```python
from build123d import *

# Parameters (mm, degrees)
Y_KSEKLIK_EKSTR_ZYON1_DEPTH = 2
Y_KSEKLIK_EKSTR_ZYON2_DEPTH = 60
IZIM3_R                     = 3.1
KES_EKSTR_ZYON1_DEPTH       = 10


with BuildPart() as part:
    # Çizim1 → Yükseklik-Ekstrüzyon1 (new body)
    with BuildSketch(Plane(origin=(0, 0, 0), x_dir=(1, 0, 0), z_dir=(0, 1, 0))):
        with BuildLine():
            Line((10, 0), (90, 0))
            ThreePointArc((90, 0), (97.071067812, 2.928932188), (100, 10))
            Line((100, 10), (100, 50))
            ThreePointArc((100, 50), (97.071067812, 57.071067812), (90, 60))
            Line((90, 60), (10, 60))
            ThreePointArc((10, 60), (2.928932188, 57.071067812), (0, 50))
            Line((0, 50), (0, 10))
            ThreePointArc((0, 10), (2.928932188, 2.928932188), (10, 0))
        make_face()
    extrude(amount=Y_KSEKLIK_EKSTR_ZYON1_DEPTH)

    # Çizim2 → Yükseklik-Ekstrüzyon2 (add)
    with BuildSketch(Plane(origin=(0, 2, 0), x_dir=(1, 0, 0), z_dir=(0, 1, 0))):
        with BuildLine():
            Line((100, 10), (100, 50))
            ThreePointArc((100, 50), (97.071067812, 57.071067812), (90, 60))
            Line((90, 60), (10, 60))
            ThreePointArc((10, 60), (2.928932188, 57.071067812), (0, 50))
            Line((0, 50), (0, 10))
            ThreePointArc((0, 10), (2.928932188, 2.928932188), (10, 0))
            Line((10, 0), (90, 0))
            ThreePointArc((90, 0), (97.071067812, 2.928932188), (100, 10))
        make_face()
        Polygon((12, 2), (88, 2), (98, 12), (98, 48), (88, 58), (12, 58), (2, 48), (2, 12), align=None, mode=Mode.SUBTRACT)
    extrude(amount=Y_KSEKLIK_EKSTR_ZYON2_DEPTH)

    # Çizim3 → Kes-Ekstrüzyon1 (cut)
    with BuildSketch(Plane.XY):
        with Locations((20, 37)):
            Circle(IZIM3_R)
        with BuildLine():
            Line((76.4, 2), (83.4, 2))
            ThreePointArc((83.4, 2), (84.107106781, 2.292893219), (84.4, 3))
            Line((84.4, 3), (84.4, 6))
            ThreePointArc((84.4, 6), (84.107106781, 6.707106781), (83.4, 7))
            Line((83.4, 7), (76.4, 7))
            ThreePointArc((76.4, 7), (75.692893219, 6.707106781), (75.4, 6))
            Line((75.4, 6), (75.4, 3))
            ThreePointArc((75.4, 3), (75.692893219, 2.292893219), (76.4, 2))
        make_face()
    extrude(amount=-KES_EKSTR_ZYON1_DEPTH, mode=Mode.SUBTRACT)


solid = part.part
```
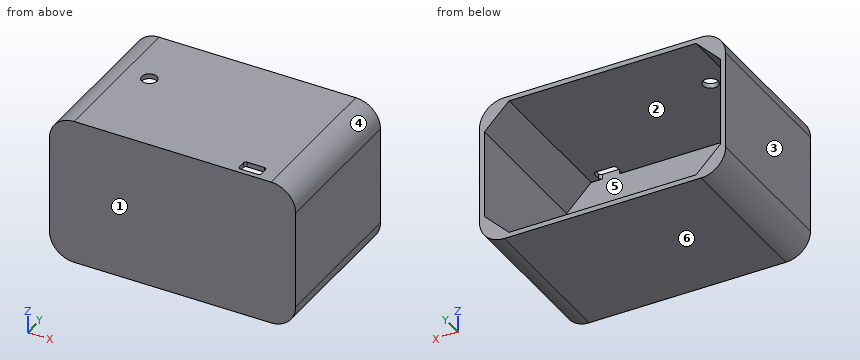
Geometry: final body of the model. Coordinates: model frame, mm. Face numbers are marked on the shaded views. A direction names the side the tool comes from. Give positions to 0.01 mm unless a question says otherwise; leave off trailing zeros. Order: outer loops, then holes, each group sorted by start corner. A loop starts at its lowest first (then second) coordinate and runs counter-clockwise, first axis right, second up. Notation, with made-up numbers: M 57,-7.5 L 105,-7.5 A18 cw 105,-2.5 Z; hole C -26,-23.5 d7. An arc over 180 degrees is marked long. Answer as CSV lines item,"result". Start each with the question number.
1) First-contact query: P1, Ø2, axis at y = 5, z = -0.5, coming from the -X side; P2, Ø1, axis at y = 5, z = -0.5, coming from the +X side; P3, Ø5, axis at x = 43, z = -11.5, coming from the +Y side. Flat tips, straight axial feed; report the tip coordinate or a pass-through.
2) Cut plane A-A (x = 20). Output: boundary loops of the cut face in (y, z).
3) Mould query, pull axis X, two halves, no side actions, for the marked faces 3, 4, 5 and 6. Classes: +X half, -X half, draft (parallel to the pull), parting line (faces both ways), or undercut.
4) Line query: line 1 (Y direction, x = 20, z = -1); line 2 (Z direction, x = 61.5, y = 6.5); line 3 (X direction, y = 7, z = -33). Output: solid intervals per line, ascending. Write a range as from..to.
5) Set-up query: the marked faces 1 and 2. Return all of +Z, -Z, +X, -X, +Y, -Y with unobstructed straight access to the full face (end or side cutting, diameter ignored); none if empty.
6) Cut plane B-B (y = 16.5). Output: boundary loops of the cut face in (x, z).
7) Cut plane C-C (x = 46). Output: boundary loops of the cut face in (y, z).
8) Cut plane D-D (y = 37). Output: boundary loops of the cut face in (x, z).
Findings below:
1,P1,"stops at x = 4.73"
1,P2,"stops at x = 94.36"
1,P3,"stops at y = 2"
2,outline,"M 0,-60 L 62,-60 L 62,-58 L 2,-58 L 2,-2 L 33.9,-2 L 33.9,0 L 0,0 Z; M 40.1,-2 L 62,-2 L 62,0 L 40.1,0 Z"
3,face 3,"-X half"
3,face 4,"+X half"
3,face 5,"undercut"
3,face 6,"draft"
4,line 1,"y = 0..33.9, 40.1..62"
4,line 2,"z = -60..-58, -2..0"
4,line 3,"x = 0..2, 98..100"
5,face 1,"+Z, -Z, +X, -X, -Y"
5,face 2,"+Y"
6,outline,"M 0,-50 A10 ccw 10,-60 L 90,-60 A10 ccw 100,-50 L 100,-10 A10 ccw 90,0 L 10,0 A10 ccw 0,-10 Z; hole M 2,-48 L 12,-58 L 88,-58 L 98,-48 L 98,-12 L 88,-2 L 12,-2 L 2,-12 Z"
7,outline,"M 0,-60 L 62,-60 L 62,-58 L 2,-58 L 2,-2 L 62,-2 L 62,0 L 0,0 Z"
8,outline,"M 0,-50 A10 ccw 10,-60 L 90,-60 A10 ccw 100,-50 L 100,-10 A10 ccw 90,0 L 23.1,0 L 23.1,-2 L 88,-2 L 98,-12 L 98,-48 L 88,-58 L 12,-58 L 2,-48 L 2,-12 L 12,-2 L 16.9,-2 L 16.9,0 L 10,0 A10 ccw 0,-10 Z"
